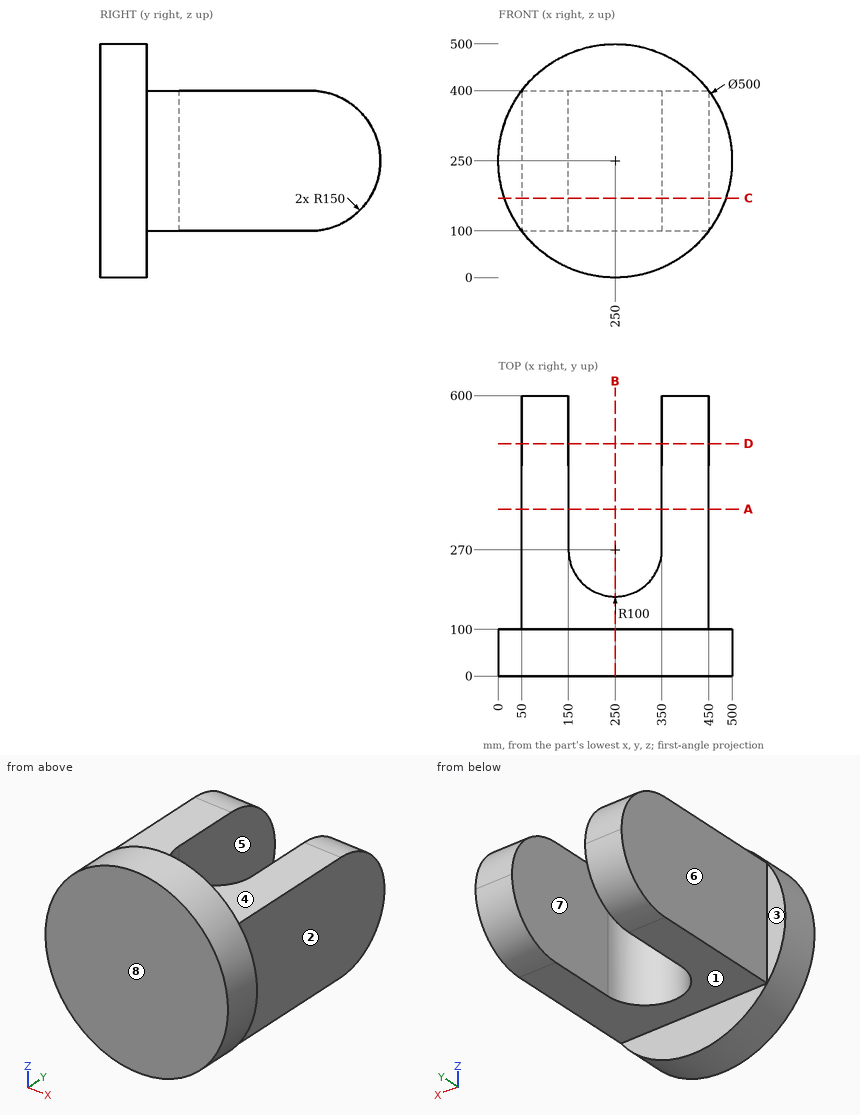
Geometry check sheet. Reference: drawing and pictorial views, mm from the part's lowest x, y, z. A direction names the side the tool comes from. Coordinates: 2 decimals unless noted, no trailing zeros. Order: outer loops, then holes, each group sorted by start corner. A loop starts at its lowest first (then second) coordinate and runs counter-clockwise, first axis right, second up. Notation, with made-up numbers: (74, 76.5) - (79, 76.5) arc R27 ccw to (79, 99.5) - close; hole circle Ø11 at (-34, -11). An arc over 180 degrees is marked (long way). One line per item, written item: value.
(1) Release check for a two-part mould opening along X. For the marked faces 5, 6, 7 and 8 record: +X half, -X half, draft (parallel to the pull), parting line (faces both ways), or undercut.
Data:
face 5: undercut
face 6: -X half
face 7: undercut
face 8: draft
(2) Sectioned sample at D-D (y = 497.5). Enter the section's corners in (x, z).
Data:
outline: (50, 107.72) - (150, 107.72) - (150, 392.28) - (50, 392.28) - close; (350, 107.72) - (450, 107.72) - (450, 392.28) - (350, 392.28) - close
(3) Depth check by flat-ended pin: pin 1 Ø1 at (x, y) = (398.5, 79.5) entering from -Z; pin 2 Ø25 at (x, z) = (485.5, 278) entering from +Y; pin 3 Ø3 at (x, y) = (406.5, 132.5) entering from -Z. Enter the tip coordinate at first touch or a pass-through.
Data:
pin 1: stops at z = 48.52
pin 2: stops at y = 100
pin 3: stops at z = 100
(4) Sectioned sample at B-B (x = 250). Enter the section's corners in (y, z), and give its area (3 significant figures).
Data:
outline: (0, 0) - (100, 0) - (100, 100) - (170, 100) - (170, 400) - (100, 400) - (100, 500) - (0, 500) - close
area: 71,000 mm^2
(5) Access from +Z, -Z, +X, -X, +Y, -Y to the whole of each face (thin tool, end or side, straight path). Record for the marked faces 1, 2, 3 and 4.
Data:
face 1: -Z, +X, -X, +Y
face 2: +Z, -Z, +X, +Y
face 3: +Z, -Z, -X, +Y
face 4: +Z, +X, -X, +Y
(6) Sectioned sample at C-C (z = 170). Enter the section's corners in (x, y).
Data:
outline: (13.15, 0) - (486.85, 0) - (486.85, 100) - (450, 100) - (450, 576.89) - (350, 576.89) - (350, 270) arc R100 cw to (150, 270) - (150, 576.89) - (50, 576.89) - (50, 100) - (13.15, 100) - close
(7) Sectioned sample at A-A (y = 357). Enter the section's corners in (x, z), and give its area (3 significant figures).
Data:
outline: (50, 100) - (150, 100) - (150, 400) - (50, 400) - close; (350, 100) - (450, 100) - (450, 400) - (350, 400) - close
area: 60,000 mm^2
(8) Thickness scan on probe 1 along X at (y, z) = (512, 215.5); probe 2 along Z at (x, y) = (75, 295.5); probe 3 along Z at (x, y) = (402.5, 455). Record the ranges inside material, lowest first. Write a range as from..to.
Data:
probe 1: x = 50..150, 350..450
probe 2: z = 100..400
probe 3: z = 100.08..399.92
